Check sheet for the modelled part. Datum: model origin and axes. Units: mm. Give positions to 0.01 mm unless a question says otherwise; leave off trailing zeros. Loops run counter-clockwise (first coordinate to the right, second up) from the corner with the lowest first, then second, coordinate; pieces in that order, holes last. Notation, with made-up numbers: (-35.5, -1.75) -> (-21.5, -1.75) arc R25 cw to (-21.5, 37.25) -> close; hole circle Ø2 at (76, 81.25). An arc over 180 degrees is marked (long way). Write each question's results on one line, items separated by ' | '. Start each with the question number.
Item 1: Cross-section at C-C on x = -1.4. Enter the section's corners in (y, z).
Item 2: Scan lines: line 1 along Y through (x, z) = (-0.9, -2); line 2 along Z through (x, y) = (-1.8, 1.4). Record each from-to range of solid material in increasing order.
Item 3: Cross-section at D-D on z = -1. Enter the section's corners in (x, y).
Item 4: Cross-section at A-A on y = 2. Enter the section's corners in (x, z).
Item 5: Mould release check, pull along Z, two halves, no side actions. Record for faces 1 (the face through (0, 3.5, 0)), 2 (the face through (0, 0, 0)): pulls with the +Z half, pulls with the -Z half, needs draft (parallel to the pull), parting line crosses it, or undercut.
Item 6: Gauge pin test, flat ends, axial feed: pin 1 Ø1.6 at (x, y) = (-1, 1) entering from -Z; pin 2 Ø1 at (x, z) = (1.5, 1) entering from -Y; pin 3 Ø0.8 at (y, z) = (1, 4) entering from -X. Record the tip position at first contact, or that the pin passes through.
Item 7: Cross-section at B-B on y = 0.6. Enter the section's corners in (x, z), then the cut area to 3 significant figures.
from build123d import *

# Parameters (mm, degrees)
EXTRUDE_1_DEPTH          = 3.5
FILLET_1_R               = 0.25
SKETCH_4_W               = 0.5
SKETCH_4_H               = 0.2
MIRROR_2_COPY_1_SKETCH_W = 0.5
MIRROR_2_COPY_1_SKETCH_H = 0.2


with BuildPart() as part:
    # Эскиз1 → Бобышка-Вытянуть1 (new body)
    with BuildSketch(Plane(origin=(0, 0, 0), x_dir=(1, 0, 0), z_dir=(0, 1, 0))):
        with BuildLine():
            Line((-2.35, -3.55), (2.35, -3.55))
            ThreePointArc((2.35, -3.55), (2.526776695, -3.476776695), (2.6, -3.3))
            Line((2.6, -3.3), (2.6, 3.3))
            ThreePointArc((2.6, 3.3), (2.526776695, 3.476776695), (2.35, 3.55))
            Line((2.35, 3.55), (-2.35, 3.55))
            ThreePointArc((-2.35, 3.55), (-2.526776695, 3.476776695), (-2.6, 3.3))
            Line((-2.6, 3.3), (-2.6, -3.3))
            ThreePointArc((-2.6, -3.3), (-2.526776695, -3.476776695), (-2.35, -3.55))
        make_face()
    extrude(amount=EXTRUDE_1_DEPTH)

    # Скругление1
    fillet_1_edges = [part.edges().sort_by_distance(p)[0] for p in [
        (2.526776695, 3.5, 3.476776695),
        (2.6, 3.5, 0),
        (2.526776695, 3.5, -3.476776695),
        (0, 3.5, -3.55),
        (-2.526776695, 3.5, -3.476776695),
        (-2.6, 3.5, 0),
        (-2.526776695, 3.5, 3.476776695),
        (0, 3.5, 3.55),
    ]]
    fillet(fillet_1_edges, radius=FILLET_1_R)

    # По траектории3: sweep along a path in Эскиз3
    with BuildLine(Plane(origin=(1.27, 0, 0), x_dir=(0, 0, -1), z_dir=(1, 0, 0))) as sweep_3_path:
        Line((-3.55, 1), (-3.86801961, 1))
        ThreePointArc((-3.86801961, 1), (-3.9314185, 0.977334214), (-3.966077677, 0.919611614))
        Line((-3.966077677, 0.919611614), (-4.133922323, 0.080388386))
        ThreePointArc((-4.133922323, 0.080388386), (-4.1685815, 0.022665786), (-4.23198039, 0))
        Line((-4.23198039, 0), (-4.6, 0))
    # Эскиз4 → По траектории3 (sweep)
    with BuildSketch(Plane.XY.offset(3.55)):
        with Locations((1.27, 1)):
            Rectangle(SKETCH_4_W, SKETCH_4_H)
    sweep_3 = sweep(path=sweep_3_path.line)

    # Зеркальное отражение1: По траектории3 across plane
    add(sweep_3.mirror(Plane.XY))

    # Зеркальное отражение2: По траектории3 across plane
    add(sweep_3.mirror(Plane(origin=(0, 0, 0), x_dir=(0, 0, 1), z_dir=(1, 0, 0))))

    # Зеркальное отражение2 copy 1: sweep along a path in Зеркальное отражение2 copy 1 path
    with BuildLine(Plane.ZY.offset(1.27)) as mirror_2_copy_1_path:
        Line((-3.55, 1), (-3.86801961, 1))
        ThreePointArc((-3.86801961, 1), (-3.9314185, 0.977334214), (-3.966077677, 0.919611614))
        Line((-3.966077677, 0.919611614), (-4.133922323, 0.080388386))
        ThreePointArc((-4.133922323, 0.080388386), (-4.1685815, 0.022665786), (-4.23198039, 0))
        Line((-4.23198039, 0), (-4.6, 0))
    # Зеркальное отражение2 copy 1 sketch → Зеркальное отражение2 copy 1 (sweep)
    with BuildSketch(Plane(origin=(0, 0, -3.55), x_dir=(-1, 0, 0), z_dir=(0, 0, -1))):
        with Locations((1.27, 1)):
            Rectangle(MIRROR_2_COPY_1_SKETCH_W, MIRROR_2_COPY_1_SKETCH_H)
    sweep(path=mirror_2_copy_1_path.line)


solid = part.part
Answer sheet:
1) outline: (-0.1, -4.6) -> (0.1, -4.6) -> (0.1, -4.23) -> (0.94, -4.06) arc R0.2 ccw to (1.1, -3.87) -> (1.1, -3.55) -> (3.25, -3.55) arc R0.25 ccw to (3.5, -3.3) -> (3.5, 3.3) arc R0.25 ccw to (3.25, 3.55) -> (1.1, 3.55) -> (1.1, 3.87) arc R0.2 ccw to (0.94, 4.06) -> (0.1, 4.23) -> (0.1, 4.6) -> (-0.1, 4.6) -> (-0.1, 4.23) arc R0.2 ccw to (0.06, 4.04) -> (0.9, 3.87) -> (0.9, 3.55) -> (0, 3.55) -> (0, -3.55) -> (0.9, -3.55) -> (0.9, -3.87) -> (0.06, -4.04) arc R0.2 ccw to (-0.1, -4.23) -> close
2) line 1: y = 0 to 3.5 | line 2: z = -3.55 to 3.55
3) outline: (-2.6, 0) -> (2.6, 0) -> (2.6, 3.25) arc R0.25 ccw to (2.35, 3.5) -> (-2.35, 3.5) arc R0.25 ccw to (-2.6, 3.25) -> close
4) outline: (-2.6, -3.3) arc R0.25 ccw to (-2.35, -3.55) -> (2.35, -3.55) arc R0.25 ccw to (2.6, -3.3) -> (2.6, 3.3) arc R0.25 ccw to (2.35, 3.55) -> (-2.35, 3.55) arc R0.25 ccw to (-2.6, 3.3) -> close
5) face 1: needs draft | face 2: undercut
6) pin 1: stops at z = -4.21 | pin 2: stops at y = 0 | pin 3: stops at x = -1.52
7) outline: (-2.6, -3.3) arc R0.25 ccw to (-2.35, -3.55) -> (2.35, -3.55) arc R0.25 ccw to (2.6, -3.3) -> (2.6, 3.3) arc R0.25 ccw to (2.35, 3.55) -> (-2.35, 3.55) arc R0.25 ccw to (-2.6, 3.3) -> close; (-1.52, -4.13) -> (-1.02, -4.13) -> (-1.02, -3.93) -> (-1.52, -3.93) -> close; (-1.52, 3.93) -> (-1.02, 3.93) -> (-1.02, 4.13) -> (-1.52, 4.13) -> close; (1.02, -4.13) -> (1.52, -4.13) -> (1.52, -3.93) -> (1.02, -3.93) -> close; (1.02, 3.93) -> (1.52, 3.93) -> (1.52, 4.13) -> (1.02, 4.13) -> close | area: 37.3 mm²
